Could you check a few things on this model? Use its own coordinates, in mm. A direction names the side the tool comes from. Coordinates: 2 decimals unless noted, no trailing zeros. Write each loop counter-clockwise with the first axis right and the second up, starting at its lowest first coordinate (ties: lowest second). Pieces come first, ordered by that corner, then holes.
```python
from build123d import *

# Parameters (mm, degrees)
BOSS_EXTRU_1_DEPTH = 2
ESQUISSE2_R        = 4
ESQUISSE2_R_2      = 1.5
BOSS_EXTRU_2_DEPTH = 6.25
ESQUISSE3_W        = 15
ESQUISSE3_H        = 7.5
BOSS_EXTRU_3_DEPTH = 10


with BuildPart() as part:
    # Esquisse1 → Boss.-Extru.1 (new body)
    with BuildSketch(Plane(origin=(0, 0, 0), x_dir=(1, 0, 0), z_dir=(0, 1, 0))):
        Polygon((-42, 45), (42, 45), (45, 42), (45, -42), (42, -45), (-42, -45), (-45, -42), (-45, 42), align=None)
    extrude(amount=BOSS_EXTRU_1_DEPTH)

    # Esquisse2 → Boss.-Extru.2 (add)
    # profile 1 of 4: a face of its own
    with BuildSketch(Plane.XZ):
        with Locations(Location((-24.5, 24.5, 0), (0, 0, 270))):
            Circle(ESQUISSE2_R)
        with Locations(Location((-24.5, 24.5, 0), (0, 0, 270))):
            Circle(ESQUISSE2_R_2, mode=Mode.SUBTRACT)
    # profile 2 of 4: a face of its own
    with BuildSketch(Plane.XZ):
        with Locations(Location((24.5, 24.5, 0), (0, 0, 270))):
            Circle(ESQUISSE2_R)
        with Locations(Location((24.5, 24.5, 0), (0, 0, 270))):
            Circle(ESQUISSE2_R_2, mode=Mode.SUBTRACT)
    # profile 3 of 4: a face of its own
    with BuildSketch(Plane.XZ):
        with Locations(Location((-24.5, -24.5, 0), (0, 0, 270))):
            Circle(ESQUISSE2_R)
        with Locations(Location((-24.5, -24.5, 0), (0, 0, 270))):
            Circle(ESQUISSE2_R_2, mode=Mode.SUBTRACT)
    # profile 4 of 4: a face of its own
    with BuildSketch(Plane.XZ):
        with Locations(Location((24.5, -24.5, 0), (0, 0, 270))):
            Circle(ESQUISSE2_R)
        with Locations(Location((24.5, -24.5, 0), (0, 0, 270))):
            Circle(ESQUISSE2_R_2, mode=Mode.SUBTRACT)
    extrude(amount=BOSS_EXTRU_2_DEPTH)

    # Esquisse3 → Boss.-Extru.3 (add)
    with BuildSketch(Plane.XZ):
        Rectangle(ESQUISSE3_W, ESQUISSE3_H)
    extrude(amount=BOSS_EXTRU_3_DEPTH)


solid = part.part
```
1. I want a section at D-D on y = -7.5. Please give me the cut outline in (x, z), plus the area to 4 significant figures.
Verdict:
outline: (-7.5, -3.75) - (7.5, -3.75) - (7.5, 3.75) - (-7.5, 3.75) - close
area: 112.5 mm2
2. On a 3-axis mill with a long thin cutter (end or side, diameter ignored), from which of +Z, -Z, +X, -X, +Y, -Y can I reach the whole of each face in a straight line? I mean faces 1 (the face through (-24, 0, -25)), 2 (the face through (-7.5, -5, 0)), 3 (the face through (1, 2, -1)). Say none if no direction works.
Verdict:
face 1: -Y
face 2: +Z, -Z, -X, -Y
face 3: +Z, -Z, +X, -X, +Y
3. I want a section at B-B on x = 0. Please give me the cut outline in (y, z).
Verdict:
outline: (-10, -3.75) - (0, -3.75) - (0, -45) - (2, -45) - (2, 45) - (0, 45) - (0, 3.75) - (-10, 3.75) - close
4. I want a section at A-A on y = -2.5. Give the number of separate pieces and of enclosed holes in the cut face, plus the area to 3 significant figures.
Verdict:
separate pieces: 5
enclosed holes: 4
area: 285 mm2
5. If we mould it in two halves opening along Z, with no side actions, what happens to faces 4 (the face through (43, 1, -44)), 5 (the face through (-23.49, -3.08, 25.61)), 6 (the face through (0, -5, 3.75))? For each: pulls with the +Z half, pulls with the -Z half, needs draft (parallel to the pull), parting line crosses it, or undercut.
Verdict:
face 4: pulls with the -Z half
face 5: undercut
face 6: pulls with the +Z half
6. I want a section at C-C on z = -24.5. Please give me the cut outline in (x, y).
Verdict:
outline: (-45, 0) - (-28.5, 0) - (-28.5, -6.25) - (-26, -6.25) - (-26, 0) - (-23, 0) - (-23, -6.25) - (-20.5, -6.25) - (-20.5, 0) - (20.5, 0) - (20.5, -6.25) - (23, -6.25) - (23, 0) - (26, 0) - (26, -6.25) - (28.5, -6.25) - (28.5, 0) - (45, 0) - (45, 2) - (-45, 2) - close
7. For pin 1 (1.5 mm diameter, centred on x = 24, z = 25, fed in from -Y); pin 2 (6 mm diameter, centred on y = -7.5, z = 1.5, fed in from -X); pin 3 (4 mm diameter, centred on x = 23.5, z = -24, fed in from -Y), each with a flat end and sliding along its axis, tell me the tip position at first contact or that it passes through.
Verdict:
pin 1: stops at y = 0
pin 2: stops at x = -7.5
pin 3: stops at y = -6.25
8. Please list where these lines run through material, in increasing order: line 1 along X through (y, z) = (-1.25, 24.5); line 2 along Y through (x, z) = (9, -1.5); line 3 along Z through (x, y) = (3.5, -7.75).
Verdict:
line 1: x = -28.5 to -26, -23 to -20.5, 20.5 to 23, 26 to 28.5
line 2: y = 0 to 2
line 3: z = -3.75 to 3.75
